Design review of the part shown in the three views and the two pictorial views. Dimensions are in mm from the part's minimum x, y and z. A direction names the side the tool comes from. Give positions to 0.01 mm unless a question says otherwise; leave off trailing zeros. Order: outer loops, then holes, each group sorted by start corner. A loop starts at its lowest first (then second) coordinate and runs counter-clockwise, first axis right, second up.
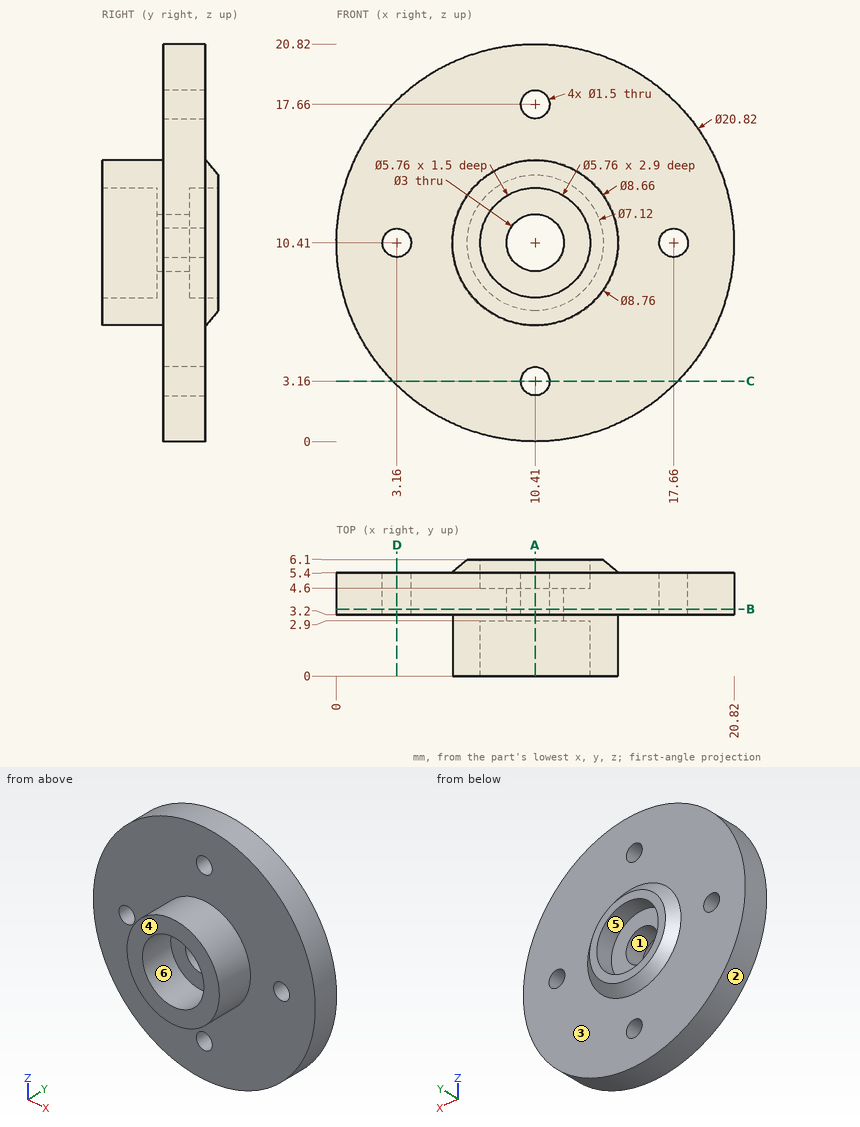
1) We need section B-B on y = 3.5. Give the boundary of the cut face in (x, z).
Answer sheet:
outline: circle Ø20.82 at (10.41, 10.41); hole circle Ø1.5 at (3.16, 10.41); hole circle Ø3 at (10.41, 10.41); hole circle Ø1.5 at (10.41, 3.16); hole circle Ø1.5 at (10.41, 17.66); hole circle Ø1.5 at (17.66, 10.41)
2) To check wall thickness, follow line 1 (X direction, y = 3.5, z = 10.41); line 2 (X direction, y = 1.95, z = 10.41); line 3 (Y direction, x = 19.25, z = 8.5). State the ranges of each line that lie inside material, in increasing order.
Answer sheet:
line 1: x = 0 to 2.41, 3.91 to 8.91, 11.91 to 16.91, 18.41 to 20.82
line 2: x = 6.08 to 7.53, 13.29 to 14.74
line 3: y = 3.2 to 5.4
3) Draft analysis for pull direction Z (two halves, no side actions). For the marked faces 1, 2 and 3, state which applies: +Z half, -Z half, draft (parallel to the pull), parting line (faces both ways), or undercut.
Answer sheet:
face 1: undercut
face 2: parting line
face 3: draft
4) We need section D-D on x = 3.16. Give the boundary of the cut face in (y, z).
Answer sheet:
outline: (3.2, 2.94) - (5.4, 2.94) - (5.4, 9.66) - (3.2, 9.66) - close; (3.2, 11.16) - (5.4, 11.16) - (5.4, 17.88) - (3.2, 17.88) - close
5) Tool access review of the marked faces 4, 5 and 6: name each direction out of +Z, -Z, +X, -X, +Y, -Y from which nothing blocks a thin tool from reaching the whole face with its end or side.
Answer sheet:
face 4: +Z, -Z, +X, -X, -Y
face 5: +Y
face 6: -Y
6) Clearance check with flat-ended pins moving along their axes: pin 1 (3 mm diameter, centred on x = 10.5, z = 9.5, fed in from +Y); pin 2 (3 mm diameter, centred on y = 4.5, z = 18, fed in from -X); pin 3 (1.5 mm diameter, centred on x = 8.5, y = 4.5, fed in from +Z). State where each tip first meets the part, or that it passes through.
Answer sheet:
pin 1: stops at y = 4.6
pin 2: stops at x = 1.97
pin 3: stops at z = 20.76
7) We need section C-C on z = 3.16. Give the boundary of the cut face in (x, y).
Answer sheet:
outline: (2.94, 3.2) - (9.66, 3.2) - (9.66, 5.4) - (2.94, 5.4) - close; (11.16, 3.2) - (17.88, 3.2) - (17.88, 5.4) - (11.16, 5.4) - close
8) We need section A-A on x = 10.41. Count the separate pieces of the cut face and the enclosed holes in it, then the cut area to 3 significant figures.
Answer sheet:
separate pieces: 4
enclosed holes: 0
area: 42.0 mm2
